from build123d import *

# Parameters (mm, degrees)
BOSS_EXTRU_1_START           = 3.85
ESQUISSE2_R                  = 41
ESQUISSE2_R_2                = 36
BOSS_EXTRU_1_DEPTH           = 3.85
ENL_V_START                  = -26.5
ESQUISSE4_R                  = 41
ESQUISSE4_R_2                = 36
ENL_V_MAT_EXTRU_2_DEPTH      = 26.5
BOSS_EXTRU_2_START           = 5
ESQUISSE5_R                  = 75
ESQUISSE5_R_2                = 36
BOSS_EXTRU_2_DEPTH           = 5
D_GAGEMENT_M81_D             = 8.4
R_P_TITION_CIRCULAIRE1_COUNT = 4


with BuildPart() as part:
    # Esquisse1 → Révolution1 (revolve)
    with BuildSketch(Plane.XY, mode=Mode.PRIVATE) as r_volution1_sk:
        Polygon((-17.5, 0.57), (-17.5, -0.57), (-36, -0.57), (-36, -50), (-41, -50), (-41, 50), (-36, 50), (-36, 0.57), align=None)
    revolve(r_volution1_sk.sketch.rotate(Axis((0, 7.711117165, 0), (0, -1, 0)), 270), axis=Axis((0, 7.711117165, 0), (0, -1, 0)))

    # Esquisse2 → Boss.-Extru.1 (add)
    with BuildSketch(Plane.XZ.offset(50).offset(BOSS_EXTRU_1_START)):
        with Locations(Location((0, 0, 0), (0, 0, 90))):
            Circle(ESQUISSE2_R)
        with Locations(Location((0, 0, 0), (0, 0, 90))):
            Circle(ESQUISSE2_R_2, mode=Mode.SUBTRACT)
    extrude(amount=-BOSS_EXTRU_1_DEPTH)

    # Esquisse4 → Enlèv. mat.-Extru.2 (cut)
    with BuildSketch(Plane(origin=(0, 50, 0), x_dir=(1, 0, 0), z_dir=(0, 1, 0)).offset(ENL_V_START)):
        with Locations(Location((0, 0, 0), (0, 0, 270))):
            Circle(ESQUISSE4_R)
        with Locations(Location((0, 0, 0), (0, 0, 270))):
            Circle(ESQUISSE4_R_2, mode=Mode.SUBTRACT)
    extrude(amount=ENL_V_MAT_EXTRU_2_DEPTH, mode=Mode.SUBTRACT)

    # Esquisse5 → Boss.-Extru.2 (add)
    with BuildSketch(Plane.XZ.offset(53.85).offset(BOSS_EXTRU_2_START)):
        with Locations(Location((0, 0, 0), (0, 0, 270))):
            Circle(ESQUISSE5_R)
        with Locations(Location((0, 0, 0), (0, 0, 90))):
            Circle(ESQUISSE5_R_2, mode=Mode.SUBTRACT)
    extrude(amount=-BOSS_EXTRU_2_DEPTH)

    # Dégagement M81 (through all)
    with Locations(Plane(origin=(0, -53.85, 0), x_dir=(1, 0, 0), z_dir=(0, 1, 0))):
        with Locations((53.123973782, -23.277530145)):
            d_gagement_m81 = Hole(D_GAGEMENT_M81_D / 2)

    # Répétition circulaire1: Dégagement M81 ×4 about axis
    r_p_tition_circulaire1_axis = Axis((0, 0, 0), (0, 1, 0))
    for i in range(1, R_P_TITION_CIRCULAIRE1_COUNT):
        add(d_gagement_m81.rotate(r_p_tition_circulaire1_axis, i * 360 / R_P_TITION_CIRCULAIRE1_COUNT), mode=Mode.SUBTRACT)


solid = part.part
Here's how the part is built. I have some questions about the finished solid (model axes, mm). A direction names the side the tool comes from. Coordinates: 2 decimals unless noted, no trailing zeros. Loops run counter-clockwise (first coordinate to the right, second up) from the corner with the lowest first, then second, coordinate; pieces in that order, holes last.
1. For P1, Ø12, axis at y = -23.5, z = -20.5, coming from the +X side; P2, Ø21.5, axis at x = 13.5, z = -17, coming from the +Y side; P3, Ø8, axis at y = 7.5, z = -11, coming from the -X side; P4, Ø21, axis at x = 0, z = 0, coming from the -Y side, each with a flat end and sliding along its axis, tell me the tip position at first contact or that it passes through.
2. Imagine slicing it at A-A, the plane x = 0. Please give me the cut outline in (y, z).
3. Imagine slicing it at B-B, the plane z = 0. Please give me the cut outline in (x, y).
4. For faces 1 (the flat face through (15.5, -0.57, 8.5)), 2 (the flat face through (-32, -53.85, -32)), 3 (the cylindrical face through (19.113, -56.385, -53.671)), which set-ups out of +Z, -Z, +X, -X, +Y, -Y let a thin tool reach every point of the face, with its end or its side?
5. I need wall thicknesses on L1, parallel to X at y = -17, z = 0; L2, parallel to Y at x = 39, z = 53. Which ranges of each line are inside material? Lowest first, please.
6. Imagine slicing it at D-D, the plane z = -31. Please give me the cut outline in (x, y), and give its area (3 significant figures).
7. Imagine slicing it at C-C, the plane y = -41. Please give me the cut outline in (x, z).
8. If we mould it in two halves opening along Z, with no side actions, what happens to faces 4 (the cylindrical face through (-45.636, -56.385, 59.517)), 5 (the cylindrical face through (-53.671, -56.385, -19.113)), 6 (the flat face through (-36.3, 23.5, -0.2))? For each: pulls with the +Z half, pulls with the -Z half, needs draft (parallel to the pull), parting line crosses it, or undercut.
Taken from the geometry:
1. P1: stops at x = 38.35
1. P2: stops at y = 0.57
1. P3: stops at x = -40.4
1. P4: passes through
2. outline: (-58.85, -75) - (-53.85, -75) - (-53.85, -41) - (23.5, -41) - (23.5, -36) - (0.57, -36) - (0.57, -17.5) - (-0.57, -17.5) - (-0.57, -36) - (-58.85, -36) - close; (-58.85, 36) - (-0.57, 36) - (-0.57, 17.5) - (0.57, 17.5) - (0.57, 36) - (23.5, 36) - (23.5, 41) - (-53.85, 41) - (-53.85, 75) - (-58.85, 75) - close
3. outline: (-75, -58.85) - (-36, -58.85) - (-36, -0.57) - (-17.5, -0.57) - (-17.5, 0.57) - (-36, 0.57) - (-36, 23.5) - (-41, 23.5) - (-41, -53.85) - (-75, -53.85) - close; (17.5, -0.57) - (36, -0.57) - (36, -58.85) - (75, -58.85) - (75, -53.85) - (41, -53.85) - (41, 23.5) - (36, 23.5) - (36, 0.57) - (17.5, 0.57) - close
4. face 1: -Y
4. face 2: +Y
4. face 3: +Y, -Y
5. L1: x = -41 to -36, 36 to 41
5. L2: y = -58.85 to -53.85
6. outline: (-68.29, -58.85) - (-18.3, -58.85) - (-18.3, -0.57) - (18.3, -0.57) - (18.3, -58.85) - (68.29, -58.85) - (68.29, -53.85) - (26.83, -53.85) - (26.83, 23.5) - (18.3, 23.5) - (18.3, 0.57) - (-18.3, 0.57) - (-18.3, 23.5) - (-26.83, 23.5) - (-26.83, -53.85) - (-68.29, -53.85) - close
6. area: 1,860 mm2
7. outline: circle Ø82 at (0, 0); hole circle Ø72 at (0, 0)
8. face 4: parting line crosses it
8. face 5: undercut
8. face 6: needs draft
